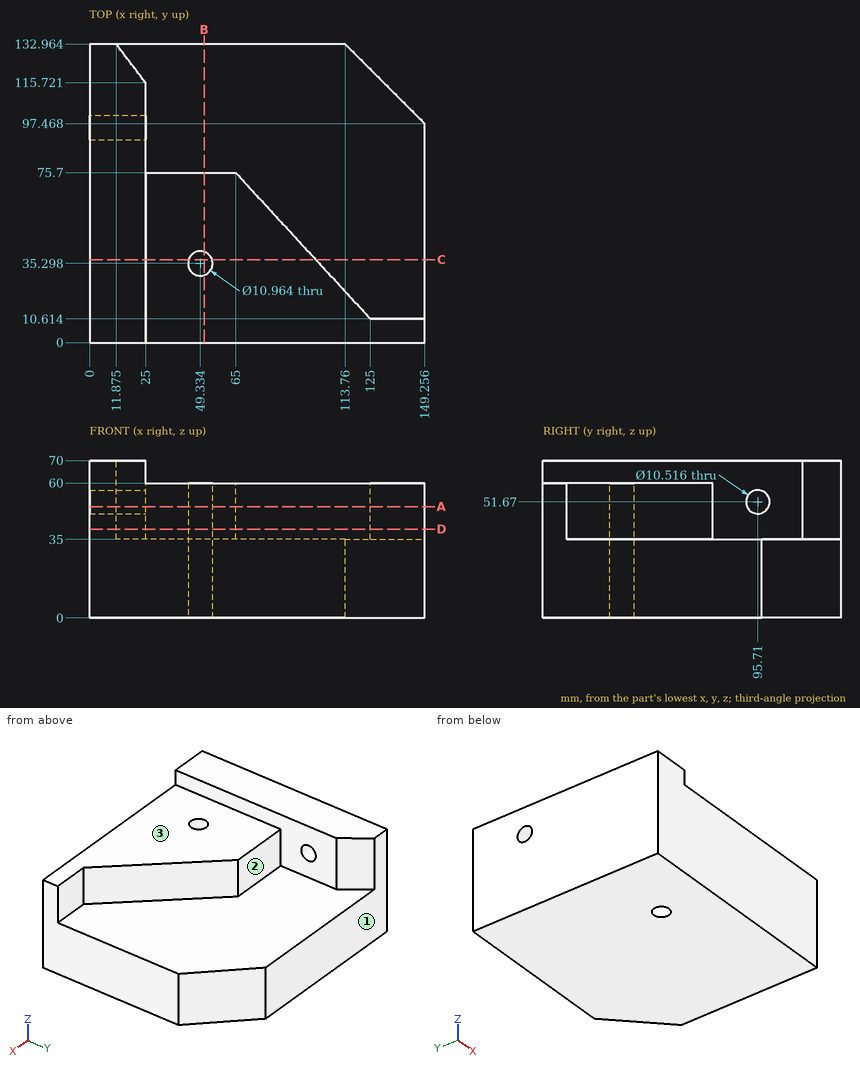
Study the drawing (mm; zero at the part's minimum x, y, z) and answer. A direction names the side the tool comes from. Coordinates: 2 decimals unless noted, no trailing zeros. Write each loop counter-clockwise with the first axis right and the second up, starting at its lowest first coordinate (ties: lowest second). Pieces come first, ordered by that corner, then holes. Notation, with made-up numbers: (19, -7.5) -> (54, -7.5) arc R30 cw to (54, 19.5) -> close; hole circle Ø9 at (-9, 36). An arc over 180 degrees is marked (long way). Write each question's results on one line, items separated by ' | '. Start each with the question number.
1) Straight lines are drawn through the part: probe 1 along Z at (x, y) = (122, 97); probe 2 along Z at (x, y) = (119, 14.5); probe 3 along X at (y, z) = (84, 50). For each, find the intervals that lie inside material, in ascending order.
2) A cutting plane is placed at C-C (y = 37). Determine the outline of the cut face in (x, z) (1 decimal).
3) A cutting plane is placed at D-D (z = 39.5). Determine the outline of the cut face in (x, y) (1 decimal), then the cut area to 3 significant figures.
4) Flat-ended cylindrical pins translate along their axes: pin 1 Ø19.5 at (x, z) = (141.5, 42.5) entering from +Y (1 decimal); pin 2 Ø6.5 at (y, z) = (95.71, 51.67) entering from +X; pin 3 Ø12 at (x, y) = (55.5, 55.5) entering from +Z; pin 4 Ø4 at (y, z) = (47, 12) entering from -X. Find the tip coordinate at first contact, or state that the pin passes through.
5) A tool of negligible diameter and unlimited length cuts with its end or side. For the marked faces 1, 2 and 3, from which of +Z, -Z, +X, -X, +Y, -Y can it reach the whole face along a straight path? Write none if from no direction.
6) A cutting plane is placed at A-A (z = 49.5). Determine the outline of the cut face in (x, y) (1 decimal).
7) A cutting plane is placed at B-B (x = 51). Determine the outline of the cut face in (y, z) (1 decimal), then the cut area to 3 significant figures.
Values follow:
1) probe 1: 0 to 35 | probe 2: 0 to 60 | probe 3: 0 to 25
2) outline: (0, 0) -> (44.1, 0) -> (44.1, 60) -> (25, 60) -> (25, 70) -> (0, 70) -> close; (54.5, 0) -> (149.3, 0) -> (149.3, 35) -> (100.7, 35) -> (100.7, 60) -> (54.5, 60) -> close
3) outline: (0, 0) -> (149.3, 0) -> (149.3, 10.6) -> (125, 10.6) -> (65, 75.7) -> (25, 75.7) -> (25, 115.7) -> (11.9, 133) -> (0, 133) -> close; hole circle Ø11 at (49.3, 35.3) | area: 8,990 mm²
4) pin 1: y = 111.5 | pin 2: through | pin 3: z = 60 | pin 4: x = 0
5) face 1: +Z, -Z, +X, -X, +Y | face 2: +Z, +X, +Y | face 3: +Z, +X, +Y, -Y
6) outline: (0, 0) -> (149.3, 0) -> (149.3, 10.6) -> (125, 10.6) -> (65, 75.7) -> (25, 75.7) -> (25, 90.9) -> (0, 90.9) -> close; (0, 100.5) -> (25, 100.5) -> (25, 115.7) -> (11.9, 133) -> (0, 133) -> close; hole circle Ø11 at (49.3, 35.3)
7) outline: (0, 0) -> (30.1, 0) -> (30.1, 60) -> (0, 60) -> close; (40.5, 0) -> (133, 0) -> (133, 35) -> (75.7, 35) -> (75.7, 60) -> (40.5, 60) -> close | area: 5,920 mm²
